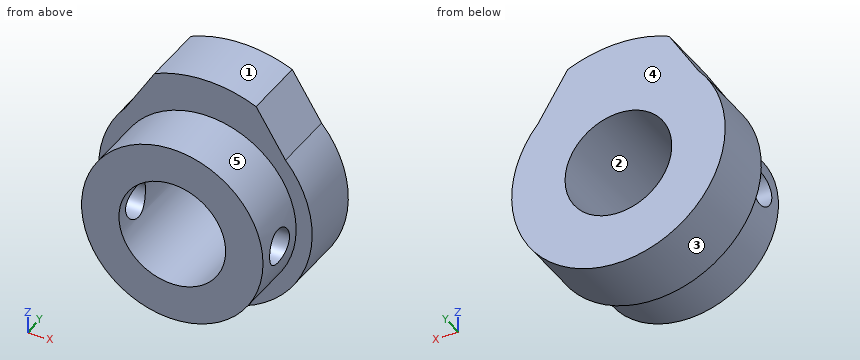
```python
from build123d import *

# Parameters (mm, degrees)
F0_R     = 8.5
F0_R_2   = 5
F1_DEPTH = 6
F2_DEPTH = 11.5
F4_D     = 3.3
F4_DEPTH = 10.001
F5_D     = 3.3


with BuildPart() as f1:
    # F0 (on Front) → F1 (new body)
    with BuildSketch(Plane.XZ):
        with BuildLine():
            Line((-4.75, 11.0198684203), (-7.5, 6.6143782777))
            ThreePointArc((-7.5, 6.6143782777), (0, -10), (7.5, 6.6143782777))
            Line((7.5, 6.6143782777), (4.75, 11.0198684203))
            ThreePointArc((4.75, 11.0198684203), (0, 12), (-4.75, 11.0198684203))
        make_face()
        Circle(F0_R, mode=Mode.SUBTRACT)
        Circle(F0_R)
        Circle(F0_R_2, mode=Mode.SUBTRACT)
    extrude(amount=F1_DEPTH)

    # F0 (on Front) → F2 (join)
    with BuildSketch(Plane.XZ):
        Circle(F0_R)
        Circle(F0_R_2, mode=Mode.SUBTRACT)
    extrude(amount=F2_DEPTH)

    # F4 (through all, one way)
    with BuildSketch(Plane(origin=(0, 0, 0), x_dir=(0, 1, 0), z_dir=(-1, 0, 0))):
        with Locations((-8.75, 0)):
            Circle(F4_D / 2)
    extrude(amount=-F4_DEPTH, mode=Mode.SUBTRACT)

    # F5 (through all)
    with Locations(Plane.YZ):
        with Locations((-8.75, 0)):
            Hole(F5_D / 2)


solid = f1.part
```
Part model, mm, in its own coordinate system. Face numbers are marked on the shaded views. A direction names the side the tool comes from. Round coordinates to 2 decimals unless told otherwise and drop trailing zeros. Write each loop counter-clockwise with the first axis right and the second up, starting at its lowest first coordinate (ties: lowest second). Pieces come first, ordered by that corner, then holes. Notation, with made-up numbers: (60, -15.75) -> (74, -15.75) arc R25 cw to (74, 22.25) -> close; hole circle Ø10 at (-37, -24.5). An arc over 180 degrees is marked (long way). Return JSON: item names as keys, results as strings. Group by question number.
Q1. Pin check, flat tips, straight feed: pin 1 (1.5 mm diameter, centred on y = -7.5, z = -4.5, fed in from -X); pin 2 (1 mm diameter, centred on x = 1.5, y = -4.5, fed in from -Z); pin 3 (4 mm diameter, centred on y = -4, z = -7.5, fed in from +X). Stop position of each tip, or through.
Q2. Saw through at B-B on x = 0. Write the cut outline in (y, z), plus the area to 4 significant figures.
Q3. Saw through at D-D on z = -3.25. Write the cut outline in (x, y), plus the area to 3 significant figures.
Q4. Saw through at A-A on z = 0. Write the cut outline in (x, y), plus the area to 3 significant figures.
Q5. Which spindle directions (+Z, -Z, +X, -X, +Y, -Y) get a long thin tool onto all of the face, cutting with end or side? Do the marked faces 4 and 5. Say none if no direction does.
Q6. Saw through at C-C on y = -8.75. Write the cut outline in (x, z), plus the area to 3 significant figures.
Q7. Probe L1, parallel to Z at x = 0, y = -7.75; L2, parallel to Y at x = 6.7, z = 0; L3, parallel to X at y = -3.5, z = 0. List the from-to ranges inside material, lowest first. Write a range as [from, to].
Q8. Mould opens along Z. For the marked faces 1, 2 and 3 say: pulls with the +Z half, pulls with the -Z half, needs draft (parallel to the pull), parting line crosses it, or undercut.
Answer:
{
 "1": {"pin 1": "x = -7.63", "pin 2": "z = -9.95", "pin 3": "x = 8.35"},
 "2": {"outline": "(-11.5, -8.5) -> (-6, -8.5) -> (-6, -10) -> (0, -10) -> (0, -5) -> (-11.5, -5) -> close; (-11.5, 5) -> (0, 5) -> (0, 12) -> (-6, 12) -> (-6, 8.5) -> (-11.5, 8.5) -> close", "area": "110.5 mm2"},
 "3": {"outline": "(-9.46, -6) -> (-7.85, -6) -> (-7.85, -11.5) -> (-3.8, -11.5) -> (-3.8, 0) -> (-9.46, 0) -> close; (3.8, -11.5) -> (7.85, -11.5) -> (7.85, -6) -> (9.46, -6) -> (9.46, 0) -> (3.8, 0) -> close", "area": "112 mm2"},
 "4": {"outline": "(-10, -6) -> (-8.5, -6) -> (-8.5, -7.1) -> (-5, -7.1) -> (-5, 0) -> (-10, 0) -> close; (-8.5, -11.5) -> (-5, -11.5) -> (-5, -10.4) -> (-8.5, -10.4) -> close; (5, -11.5) -> (8.5, -11.5) -> (8.5, -10.4) -> (5, -10.4) -> close; (5, -7.1) -> (8.5, -7.1) -> (8.5, -6) -> (10, -6) -> (10, 0) -> (5, 0) -> close", "area": "75.4 mm2"},
 "5": {"face 4": "+Z, -Z, +X, -X, +Y", "face 5": "-Y"},
 "6": {"outline": "(-8.34, -1.65) arc R8.5 ccw to (8.34, -1.65) -> (4.72, -1.65) arc R5 cw to (-4.72, -1.65) -> close; (-8.34, 1.65) -> (-4.72, 1.65) arc R5 cw to (4.72, 1.65) -> (8.34, 1.65) arc R8.5 ccw to start", "area": "125 mm2"},
 "7": {"L1": "[-8.5, -5], [5, 8.5]", "L2": "[-11.5, -10.4], [-7.1, 0]", "L3": "[-10, -5], [5, 10]"},
 "8": {"face 1": "pulls with the +Z half", "face 2": "undercut", "face 3": "parting line crosses it"}
}
